from build123d import *

# Parameters (mm, degrees)
HOLE_D             = 8.7
HOLE_DEPTH         = 25
HOLE_CSINK_D       = 14.79
HOLE_CSINK_ANGLE   = 82
POLARPATTERN_COUNT = 4


with BuildPart() as part:
    # Sketch → Revolution (revolve)
    with BuildSketch(Plane.XZ):
        Polygon((14.86, 0), (47.625, 0), (47.625, 8), (22.86, 8), (22.86, 17.78), (14.86, 17.78), align=None)
    revolve(axis=Axis((0, 0, 0), (0, 0, 1)))

    # Hole
    with Locations(Plane.XY.offset(8)):
        with Locations((0, 35)):
            hole = CounterSinkHole(HOLE_D / 2, HOLE_CSINK_D / 2, depth=HOLE_DEPTH, counter_sink_angle=HOLE_CSINK_ANGLE)

    # PolarPattern: Hole ×4 about axis
    polarpattern_axis = Axis((0, 0, 8), (0, 0, 1))
    for i in range(1, POLARPATTERN_COUNT):
        add(hole.rotate(polarpattern_axis, i * 360 / POLARPATTERN_COUNT), mode=Mode.SUBTRACT)


solid = part.part
Read the model definition and answer for the solid it produces. Units are mm, in the model's axes. A direction names the side the tool comes from. Coordinates: 2 decimals unless noted, no trailing zeros. Write each loop counter-clockwise with the first axis right and the second up, starting at its lowest first coordinate (ties: lowest second). Pieces come first, ordered by that corner, then holes. Notation, with made-up numbers: (-40, 75.5) -> (15, 75.5) arc R36 ccw to (15, 112.5) -> close; hole circle Ø3 at (19, 89). An arc over 180 degrees is marked (long way). Return JSON: item names as keys, results as strings.
(1) The part is cut by section D-D on z = 2.25. Give the vertices of the cut face in (x, y) (3 decimals).
Answers below:
{"outline": "circle Ø95.25 at (0, 0); hole circle Ø8.7 at (-35, 0); hole circle Ø29.72 at (0, 0); hole circle Ø8.7 at (0, -35); hole circle Ø8.7 at (0, 35); hole circle Ø8.7 at (35, 0)"}
(2) Consider line 1 along Y through (x, z) = (0, 3.6) (3 decimals); line 2 along Y through (x, z) = (0, 9.5); line 3 along Z through (x, y) = (-24.5, -29). Determine where each line is inside the solid, lowest interval first. Write a range as from..to.
Answers below:
{"line 1": "-47.625..-39.35, -30.65..-14.86, 14.86..30.65, 39.35..47.625", "line 2": "-22.86..-14.86, 14.86..22.86", "line 3": "0..8"}
(3) The part is cut by section A-A on y = 0. Give the vertices of the cut face in (x, z) (3 decimals), then the cut area to 3 significant figures.
Answers below:
{"outline": "(-47.625, 0) -> (-39.35, 0) -> (-39.35, 4.497) -> (-42.395, 8) -> (-47.625, 8) -> close; (-30.65, 0) -> (-14.86, 0) -> (-14.86, 17.78) -> (-22.86, 17.78) -> (-22.86, 8) -> (-27.605, 8) -> (-30.65, 4.497) -> close; (14.86, 0) -> (30.65, 0) -> (30.65, 4.497) -> (27.605, 8) -> (22.86, 8) -> (22.86, 17.78) -> (14.86, 17.78) -> close; (39.35, 0) -> (47.625, 0) -> (47.625, 8) -> (42.395, 8) -> (39.35, 4.497) -> close", "area": "520 mm^2"}
(4) Each of these flat-tipped pins is pushed along its axis until it touches: P1, Ø6, axis at x = 13, z = 4, coming from the -Y side; P2, Ø2, axis at x = 34, z = 6.5, coming from the -Y side; P3, Ø4, axis at x = -7, y = 34, coming from the -Z side; P4, Ø4, axis at x = -37, z = 8.5, coming from the +Y side. Where does it stop, or does it pass through?
Answers below:
{"P1": "y = -46.56", "P2": "y = -34.34", "P3": "z = 0", "P4": "y = 32.23"}
(5) Which of the six approach directions +Z, -Z, +X, -X, +Y, -Y give full straight-line access (tool end or side, diameter ignored) to faces 5 (the flat face through (20.5, 11.3, 8)), 6 (the cylindrical face through (-10.952, 10.043, 8.766))?
Answers below:
{"face 5": "+Z", "face 6": "+Z, -Z"}
(6) The part is cut by section C-C on y = 12.5. Give the vertices of the cut face in (x, z), then the cut area to 3 significant figures.
Answers below:
{"outline": "(-45.96, 0) -> (-8.04, 0) -> (-8.04, 17.78) -> (-19.14, 17.78) -> (-19.14, 8) -> (-45.96, 8) -> close; (8.04, 0) -> (45.96, 0) -> (45.96, 8) -> (19.14, 8) -> (19.14, 17.78) -> (8.04, 17.78) -> close", "area": "824 mm^2"}
(7) For a pull along X with two mould halves and no side action, classify faces 1 (the cylindrical face through (39.313, -0.566, 2.217)), 2 (the cylindrical face through (-39.313, 0.566, 2.217)), 3 (the cylindrical face through (21.804, 6.867, 12.958)), 4 (the flat face through (5, -15, 17.78)) as pulls with the +X half, pulls with the -X half, needs draft (parallel to the pull), parting line crosses it, or undercut.
Answers below:
{"face 1": "undercut", "face 2": "undercut", "face 3": "parting line crosses it", "face 4": "needs draft"}
(8) The part is cut by section B-B on x = 10.5. Give the vertices of the cut face in (y, z), then the cut area to 3 significant figures.
Answers below:
{"outline": "(-46.45, 0) -> (-10.52, 0) -> (-10.52, 17.78) -> (-20.31, 17.78) -> (-20.31, 8) -> (-46.45, 8) -> close; (10.52, 0) -> (46.45, 0) -> (46.45, 8) -> (20.31, 8) -> (20.31, 17.78) -> (10.52, 17.78) -> close", "area": "767 mm^2"}
